For this review, take the finished solid that the model builds, in its own axes (mm). Face numbers are marked on the shaded views. Give positions to 0.01 mm unless a question says otherwise; leave off trailing zeros. Write each loop counter-clockwise with the first axis right and the second up, starting at its lowest first coordinate (ties: lowest second). Pieces come first, ordered by that corner, then holes. Notation, with made-up numbers: (50, 43.25) -> (75, 43.25) arc R13 ccw to (75, 52.25) -> close; hole circle Ø7 at (-38.5, 44.25). An arc over 180 degrees is marked (long way). Answer as CSV lines item,"result".
```python
from build123d import *

# Parameters (mm, degrees)
ESQUISSE1_W             = 400
ESQUISSE1_H             = 222
BOSS_EXTRU_1_DEPTH      = 292
ESQUISSE2_W             = 356
ESQUISSE2_H             = 270
ENL_V_MAT_EXTRU_1_DEPTH = 428.684801456
ESQUISSE8_W             = 270
ESQUISSE8_H             = 156
ENL_V_MAT_EXTRU_2_DEPTH = 513.128650853
ESQUISSE9_W             = 356
ESQUISSE9_H             = 178
ENL_V_MAT_EXTRU_3_DEPTH = 389.126325339
ESQUISSE10_W            = 22
ESQUISSE10_H            = 22
ENL_V_MAT_EXTRU_4_DEPTH = 400
ESQUISSE11_W            = 22
ESQUISSE11_H            = 200
BOSS_EXTRU_2_DEPTH      = 400
BOSS_EXTRU_3_DEPTH      = 22
BOSS_EXTRU_4_DEPTH      = 22


with BuildPart() as part:
    # Esquisse1 → Boss.-Extru.1 (new body)
    with BuildSketch(Plane.XY):
        with Locations((19.923371648, -19.429118774)):
            Rectangle(ESQUISSE1_W, ESQUISSE1_H)
    extrude(amount=BOSS_EXTRU_1_DEPTH)

    # Esquisse2 → Enlèv. mat.-Extru.1 (cut, through all)
    with BuildSketch(Plane.XZ.offset(130.429118774)):
        with Locations((19.923371648, 135)):
            Rectangle(ESQUISSE2_W, ESQUISSE2_H)
    extrude(amount=-ENL_V_MAT_EXTRU_1_DEPTH, mode=Mode.SUBTRACT)

    # Esquisse8 → Enlèv. mat.-Extru.2 (cut, through all)
    with BuildSketch(Plane(origin=(219.923371648, 0, 0), x_dir=(0, 0, -1), z_dir=(1, 0, 0))):
        with Locations((-135, -8.429118774)):
            Rectangle(ESQUISSE8_W, ESQUISSE8_H)
    extrude(amount=-ENL_V_MAT_EXTRU_2_DEPTH, mode=Mode.SUBTRACT)

    # Esquisse9 → Enlèv. mat.-Extru.3 (cut, through all)
    with BuildSketch(Plane.XY.offset(292)):
        with Locations((19.923371648, -19.429118774)):
            Rectangle(ESQUISSE9_W, ESQUISSE9_H)
    extrude(amount=-ENL_V_MAT_EXTRU_3_DEPTH, mode=Mode.SUBTRACT)

    # Esquisse10 → Enlèv. mat.-Extru.4 (cut)
    with BuildSketch(Plane(origin=(219.923371648, 0, 0), x_dir=(0, 0, -1), z_dir=(1, 0, 0))):
        with Locations((-11, -119.429118774)):
            Rectangle(ESQUISSE10_W, ESQUISSE10_H)
    extrude(amount=-ENL_V_MAT_EXTRU_4_DEPTH, mode=Mode.SUBTRACT)

    # Esquisse11 → Boss.-Extru.2 (add)
    with BuildSketch(Plane(origin=(219.923371648, 0, 0), x_dir=(0, 0, -1), z_dir=(1, 0, 0))):
        with Locations((-11, -8.429118774)):
            Rectangle(ESQUISSE11_W, ESQUISSE11_H)
    extrude(amount=-BOSS_EXTRU_2_DEPTH)

    # Esquisse12 → Boss.-Extru.3 (add)
    with BuildSketch(Plane(origin=(219.923371648, 0, 0), x_dir=(0, 0, -1), z_dir=(1, 0, 0))):
        Polygon((70, -108.429118774), (0, 91.570881226), (0, -108.429118774), align=None)
    extrude(amount=-BOSS_EXTRU_3_DEPTH)

    # Esquisse13 → Boss.-Extru.4 (add)
    with BuildSketch(Plane.ZY.offset(180.076628352)):
        Polygon((0, -108.429118774), (-70, -108.429118774), (0, 91.570881226), align=None)
    extrude(amount=-BOSS_EXTRU_4_DEPTH)


solid = part.part
```
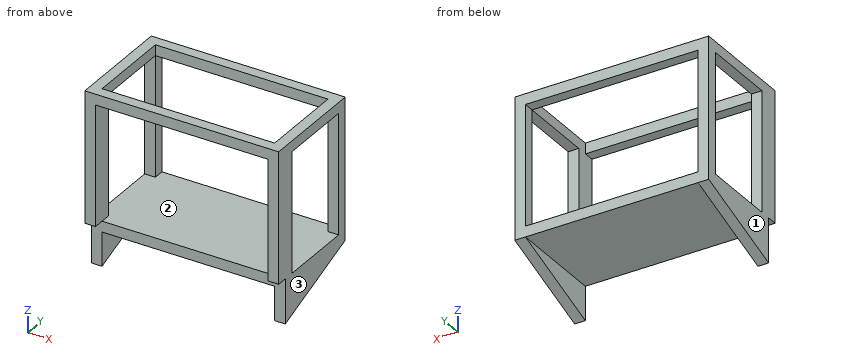
Q1. Add section A-A (z = 203). Write out the cut boundary in (x, y).
Answer block:
outline,"(-180.08, -130.43) -> (-158.08, -130.43) -> (-158.08, -86.43) -> (-180.08, -86.43) -> close; (-180.08, 69.57) -> (-158.08, 69.57) -> (-158.08, 91.57) -> (-180.08, 91.57) -> close; (197.92, -130.43) -> (219.92, -130.43) -> (219.92, -86.43) -> (197.92, -86.43) -> close; (197.92, 69.57) -> (219.92, 69.57) -> (219.92, 91.57) -> (197.92, 91.57) -> close"
Q2. To check wall thickness, follow probe 1 along Z at (x, y) = (30, 70.5); probe 2 along X at (y, z) = (-115, 52.5); probe 3 along Z at (x, y) = (-32, 67.5). State the ranges of each line that lie inside material, in increasing order. Write a range as [from, to].
Answer block:
probe 1,"z = [0, 22], [270, 292]"
probe 2,"x = [-180.08, -158.08], [197.92, 219.92]"
probe 3,"z = [0, 22]"
Q3. Add section C-C (y = -0.5). Write out the cut boundary in (x, z).
Answer block:
outline,"(-180.08, -32.22) -> (-158.08, -32.22) -> (-158.08, 0) -> (197.92, 0) -> (197.92, -32.22) -> (219.92, -32.22) -> (219.92, 22) -> (-180.08, 22) -> close; (-180.08, 270) -> (-158.08, 270) -> (-158.08, 292) -> (-180.08, 292) -> close; (197.92, 270) -> (219.92, 270) -> (219.92, 292) -> (197.92, 292) -> close"
Q4. Draft analysis for pull direction X (two halves, no side actions). For the marked faces 1, 2 and 3, state which applies: released by +X, released by -X, zero draft, split by the parting line, or undercut.
Answer block:
face 1,"released by -X"
face 2,"undercut"
face 3,"released by +X"
Q5. Add section B-B (x = 87). Write out the cut boundary in (y, z), plus the area to 3 significant figures.
Answer block:
outline,"(-130.43, 270) -> (-108.43, 270) -> (-108.43, 292) -> (-130.43, 292) -> close; (-108.43, 0) -> (91.57, 0) -> (91.57, 22) -> (-108.43, 22) -> close; (69.57, 270) -> (91.57, 270) -> (91.57, 292) -> (69.57, 292) -> close"
area,"5,370 mm2"
Q6. Clearance check with flat-ended pins moving along their axes: pin 1 (17.5 mm diameter, centred on x = -52, y = -118, fed in from -Z); pin 2 (24 mm diameter, centred on x = -164.5, y = -121, fed in from -Z); pin 3 (1 mm diameter, centred on x = -139, y = -1.5, fed in from +Z). State where each tip first meets the part, or that it passes through.
Answer block:
pin 1,"stops at z = 270"
pin 2,"stops at z = 22"
pin 3,"stops at z = 22"
Q7. Add section D-D (z = -31.5). Write out the cut boundary in (x, y).
Answer block:
outline,"(-180.08, -108.43) -> (-158.08, -108.43) -> (-158.08, 1.57) -> (-180.08, 1.57) -> close; (197.92, -108.43) -> (219.92, -108.43) -> (219.92, 1.57) -> (197.92, 1.57) -> close"
